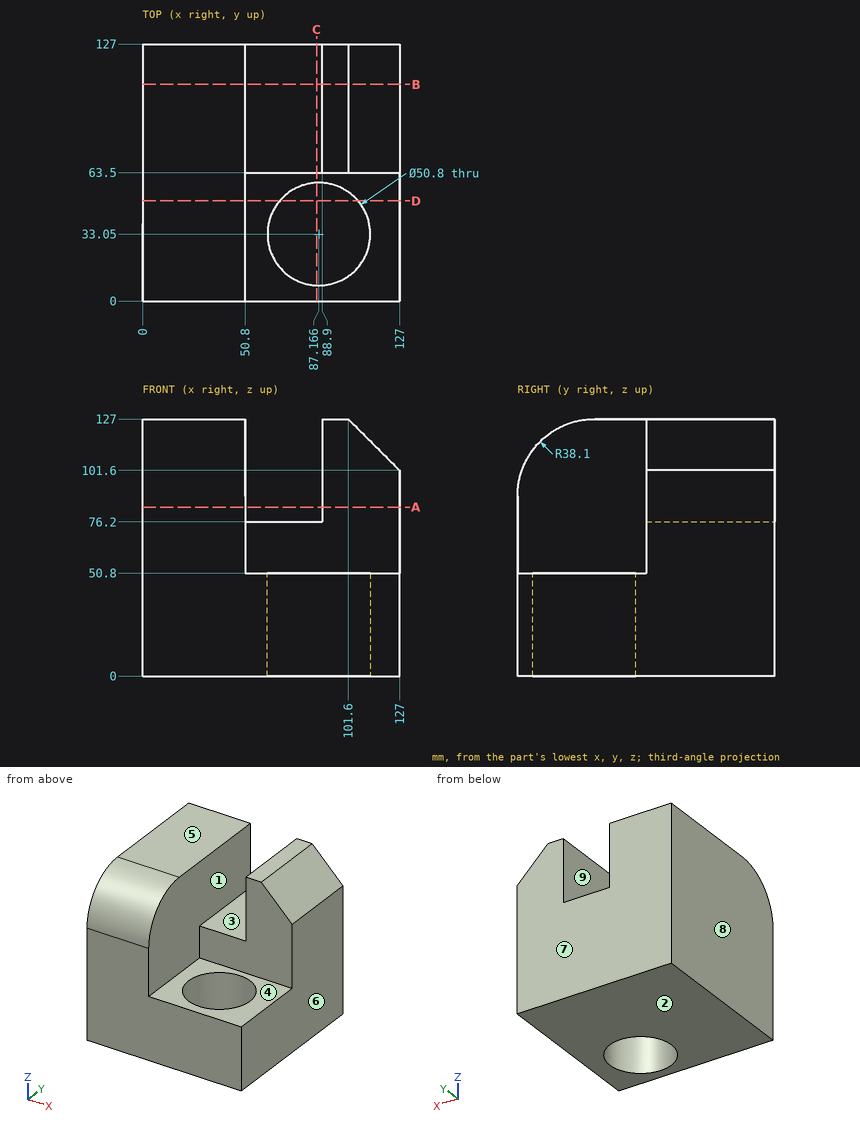
Study the drawing (mm; zero at the part's minimum x, y, z) and answer. A direction names the side the tool comes from. Give positions to 0.01 mm unless a question says otherwise; leave off trailing zeros. Write each loop counter-clockwise with the first axis right and the second up, starting at its lowest first coordinate (ties: lowest second). Pieces come first, ordered by that corner, then holes. Notation, with made-up numbers: (52.5, 34.25) - (61.5, 34.25) arc R16 cw to (61.5, 55.25) - close; hole circle Ø7 at (41.25, 33). An arc over 180 degrees is marked (long way). One line per question, with ' | ' between items. Start each with the question number.
1. Section D-D, the plane y = 49.5 is taken. Determine the outline of the cut face in (x, z), then the cut area to 3 significant figures.
2. Given P1, Ø1, axis at y = 51.5, z = 81, coming from the +X side; P2, Ø5, axis at x = 82.5, z = 77, coming from the -Y side; P3, Ø19, axis at x = 73, y = 111, coming from the +Z side, each flat-ended and moving along its own axis, determine where each tip first touches the part or whether it passes through.
3. Section A-A, the plane z = 83.5 is taken. Determine the outline of the cut face in (x, y).
4. Section C-C, the plane x = 86 is taken. Determine the outline of the cut face in (y, z).
5. Section B-B, the plane y = 107 is taken. Determine the outline of the cut face in (x, z).
6. Determine the mould class of the marked faces 6, 7, 8 and 9 for opening direction X: +X half, -X half, draft (parallel to the pull), parting line (faces both ways), or undercut.
7. Straight lines are drawn through the part: line 1 (Y direction, x = 88.5, z = 20) (1 decimal); line 2 (Y direction, x = 117.5, z = 70); line 3 (X direction, y = 49.5, z = 81). For each, find the intervals that lie inside material, in ascending order.
8. For the marked faces 1, 2, 3, 4 and 5, determine the directions among +Z, -Z, +X, -X, +Y, -Y from which every point of the face is accessible in a straight line to the end or side of a thin tool.
Result:
1) outline: (0, 0) - (67.81, 0) - (67.81, 50.8) - (50.8, 50.8) - (50.8, 127) - (0, 127) - close; (106.52, 0) - (127, 0) - (127, 50.8) - (106.52, 50.8) - close | area: 8,360 mm2
2) P1: stops at x = 50.8 | P2: stops at y = 63.5 | P3: stops at z = 76.2
3) outline: (0, 0) - (50.8, 0) - (50.8, 127) - (0, 127) - close; (88.9, 63.5) - (127, 63.5) - (127, 127) - (88.9, 127) - close
4) outline: (0, 0) - (7.68, 0) - (7.68, 50.8) - (0, 50.8) - close; (58.42, 0) - (127, 0) - (127, 76.2) - (63.5, 76.2) - (63.5, 50.8) - (58.42, 50.8) - close
5) outline: (0, 0) - (127, 0) - (127, 101.6) - (101.6, 127) - (88.9, 127) - (88.9, 76.2) - (50.8, 76.2) - (50.8, 127) - (0, 127) - close
6) face 6: +X half | face 7: draft | face 8: -X half | face 9: undercut
7) line 1: y = 0 to 7.7, 58.4 to 127 | line 2: y = 63.5 to 127 | line 3: x = 0 to 50.8
8) face 1: +Z, -Y | face 2: -Z, +X, -X, +Y, -Y | face 3: +Z, +Y, -Y | face 4: +Z, +X, -Y | face 5: +Z, +X, -X, +Y, -Y
